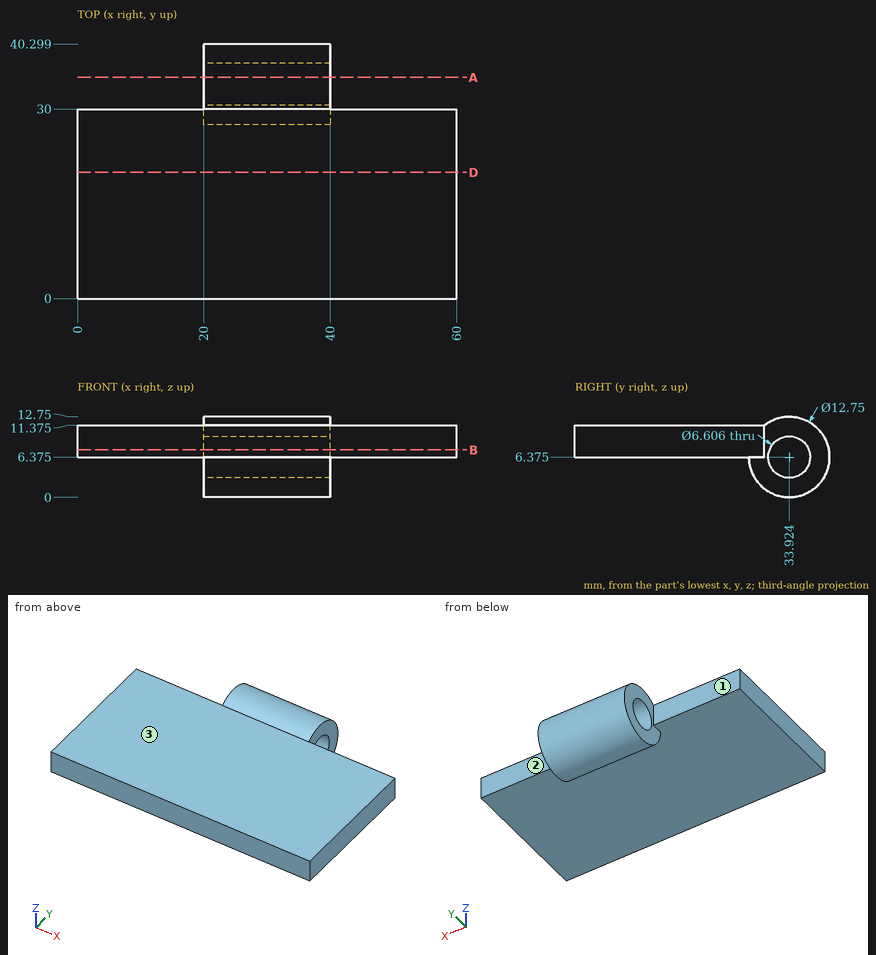
Design review of the part shown in the three views and the two pictorial views. Dimensions are in mm from the part's minimum x, y and z. A direction names the side the tool comes from. Coordinates: 2 decimals unless noted, no trailing zeros. Write each loop counter-clockwise with the first axis right and the second up, starting at its lowest first coordinate (ties: lowest second). Pieces come first, ordered by that corner, then holes.
1) To check wall thickness, follow probe 1 along Z at (x, y) = (7, 26.5) (1 decimal); probe 2 along Z at (x, y) = (35, 36) (1 decimal); probe 3 along Y at (x, z) = (24.5, 8). State the ranges of each line that lie inside material, in increasing order.
2) We need section A-A on y = 35. State the section outline as (x, z) points, then the cut area to 3 significant figures.
3) We need section B-B on z = 7.5. State the section outline as (x, y) points, then the cut area to 3 significant figures.
4) Clearance check with flat-ended pins moving along their axes: pin 1 Ø2 at (x, y) = (29.5, 31.5) entering from +Z; pin 2 Ø24 at (x, y) = (25.5, 8) entering from -Z (3 decimals); pin 3 Ø5.5 at (x, z) = (53, 8) entering from +Y. State where each tip first meets the part, or that it passes through.
5) Machinability: for the marked faces 1, 2 and 3, which of the approach directions +Z, -Z, +X, -X, +Y, -Y give a long, thin tool a straight path to every point of the face, cutting with its end or side? Answer none if there is none.
6) We need section D-D on y = 20. State the section outline as (x, z) points (1 decimal).
Answer list:
1. probe 1: z = 6.4 to 11.4
1. probe 2: z = 0.3 to 3.8, 8.9 to 12.4
1. probe 3: y = 0 to 31.05, 36.8 to 40.09
2. outline: (20, 0.09) - (40, 0.09) - (40, 3.25) - (20, 3.25) - close; (20, 9.5) - (40, 9.5) - (40, 12.66) - (20, 12.66) - close
2. area: 126 mm2
3. outline: (0, 0) - (60, 0) - (60, 30) - (40, 30) - (40, 30.82) - (20, 30.82) - (20, 30) - (0, 30) - close; (20, 37.03) - (40, 37.03) - (40, 40.2) - (20, 40.2) - close
3. area: 1,880 mm2
4. pin 1: stops at z = 12.59
4. pin 2: stops at z = 6.375
4. pin 3: stops at y = 30
5. face 1: +Z, -Z, -X, +Y
5. face 2: +Z, -Z, +X, +Y
5. face 3: +Z, +X, -X, -Y
6. outline: (0, 6.4) - (60, 6.4) - (60, 11.4) - (0, 11.4) - close
